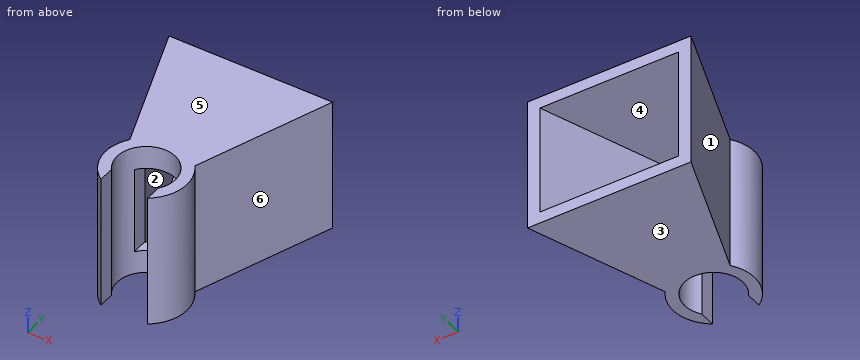
```python
from build123d import *

# Parameters (mm, degrees)
F1_DEPTH = 23
F3_DEPTH = 2
F5_DEPTH = 2
F6_W     = 8
F6_H     = 15
F7_DEPTH = 25


with BuildPart() as f1:
    # F0 (on Top) → F1 (new body)
    with BuildSketch(Plane.XY):
        with BuildLine():
            Line((-14.0209387689, 27.4292568356), (-5.5771887097, 4.2302442124))
            ThreePointArc((-5.5771887097, 4.2302442124), (-4.8480847739, 5.0493637247), (-4, 5.7445626465))
            Line((-4, 5.7445626465), (-11.892583224, 27.4292568356))
            Line((-11.892583224, 27.4292568356), (-14.0209387689, 27.4292568356))
        make_face()
        with BuildLine():
            ThreePointArc((-4, -3), (0, 5), (4, -3))
            Line((4, -3), (4, -5.7445626465))
            ThreePointArc((4, -5.7445626465), (6.9141036197, -1.0932388287), (5.5771887097, 4.2302442124))
            ThreePointArc((5.5771887097, 4.2302442124), (4.8480847739, 5.0493637247), (4, 5.7445626465))
            ThreePointArc((4, 5.7445626465), (0, 7), (-4, 5.7445626465))
            ThreePointArc((-4, 5.7445626465), (-4.8480847739, 5.0493637247), (-5.5771887097, 4.2302442124))
            ThreePointArc((-5.5771887097, 4.2302442124), (-6.9141036197, -1.0932388287), (-4, -5.7445626465))
            Line((-4, -5.7445626465), (-4, -3))
        make_face()
        with BuildLine():
            ThreePointArc((4, 5.7445626465), (4.8480847739, 5.0493637247), (5.5771887097, 4.2302442124))
            Line((5.5771887097, 4.2302442124), (14.0209387689, 27.4292568356))
            Line((14.0209387689, 27.4292568356), (11.892583224, 27.4292568356))
            Line((11.892583224, 27.4292568356), (4, 5.7445626465))
        make_face()
    extrude(amount=F1_DEPTH)

    # F2 (on face) → F3 (join)
    with BuildSketch(Plane.XY.offset(23)):
        with BuildLine():
            Line((11.892583224, 27.4292568356), (-11.892583224, 27.4292568356))
            Line((-11.892583224, 27.4292568356), (-4, 5.7445626465))
            ThreePointArc((-4, 5.7445626465), (0, 7), (4, 5.7445626465))
            Line((4, 5.7445626465), (11.892583224, 27.4292568356))
        make_face()
    extrude(amount=-F3_DEPTH)

    # F4 (on face) → F5 (join)
    with BuildSketch(Plane(origin=(0, 0, 0), x_dir=(1, 0, 0), z_dir=(0, 0, -1))):
        with BuildLine():
            Line((-11.892583224, -27.4292568356), (11.892583224, -27.4292568356))
            Line((11.892583224, -27.4292568356), (4, -5.7445626465))
            ThreePointArc((4, -5.7445626465), (0, -7), (-4, -5.7445626465))
            Line((-4, -5.7445626465), (-11.892583224, -27.4292568356))
        make_face()
    extrude(amount=-F5_DEPTH)

    # F6 (on Front) → F7 (cut)
    with BuildSketch(Plane.XZ):
        with Locations((0, 11.5)):
            Rectangle(F6_W, F6_H)
    extrude(amount=-F7_DEPTH, mode=Mode.SUBTRACT)


solid = f1.part
```
For this review, take the finished solid that the model builds, in its own axes (mm). Face numbers are marked on the shaded views. A direction names the side the tool comes from. Give positions to 0.01 mm unless a question says otherwise; leave off trailing zeros. Write each loop counter-clockwise with the first axis right and the second up, starting at its lowest first coordinate (ties: lowest second). Pieces come first, ordered by that corner, then holes. Notation, with made-up numbers: M -28.75,-14.5 L 8.25,-14.5 A28 cw 8.25,7.5 Z; hole C 79.5,89.25 d7. An arc over 180 degrees is marked long. One line per item, written item: value.
1) Take a section at B-B, the plane x = 0. Write out the cut boundary in (y, z).
Results are:
outline: M 5,0 L 27.43,0 L 27.43,2 L 7,2 L 7,4 L 5,4 Z; M 5,19 L 7,19 L 7,21 L 27.43,21 L 27.43,23 L 5,23 Z
2) Take a section at C-C, the plane z = 13.5. Write out the cut boundary in (x, y), then the cut area to 3 significant figures.
Results are:
outline: M -14.02,27.43 L -5.58,4.23 A7 ccw -4,-5.74 L -4,-3 A5 cw -4,3 L -4,5.74 L -11.89,27.43 Z; M 4,-5.74 A7 ccw 5.58,4.23 L 14.02,27.43 L 11.89,27.43 L 4,5.74 L 4,3 A5 cw 4,-3 Z
area: 135 mm²
3) For the marked faces 4, 5 and 6, list the 3-axis set-ups (+Z, -Z, +X, -X, +Y, -Y) from which the entire face can be reached by the end or side of a thin tool; tool diameter is ignored.
Results are:
face 4: +Y
face 5: +Z, +X, -X, +Y, -Y
face 6: +Z, -Z, +X
4) Take a section at A-A, the plane y = 0. Write out the cut boundary in (x, z), then the cut area to 3 significant figures.
Results are:
outline: M -7,0 L -5,0 L -5,23 L -7,23 Z; M 5,0 L 7,0 L 7,23 L 5,23 Z
area: 92.0 mm²
5) For line 1 (X direction, y = 4, z = 2.25); line 2 (X direction, y = 0, z = 5.25); line 3 (Z direction, x = 4.75, y = 26), list the stretches that pass through material, from the lowest coordinate up. Write a range as from..to.
Results are:
line 1: x = -5.74..-3, 3..5.74
line 2: x = -7..-5, 5..7
line 3: z = 0..2, 21..23
6) The part is to be moulded in two halves that separate along Z. For the marked faces 1, 2 and 3, say which applies: +Z half, -Z half, draft (parallel to the pull), parting line (faces both ways), or undercut.
Results are:
face 1: draft
face 2: undercut
face 3: -Z half
7) For P1, Ø8, axis at y = 23.5, z = 3.5, coming from the -X side; P2, Ø2, axis at y = -4, z = 17, coming from the +X side; P3, Ø0.8, axis at y = 4, z = 10, coming from the +X side; P4, Ø8, axis at x = 0, y = 0, coming from the -Z side, all flat-tipped, find the tip position at first contact; note any pin that passes through.
Results are:
P1: stops at x = -14.02
P2: stops at x = 6.32
P3: stops at x = 6
P4: passes through
8) Take a section at D-D, the plane z = 1.5. Write out the cut boundary in (x, y).
Results are:
outline: M -14.02,27.43 L -5.58,4.23 A7 ccw -4,-5.74 L -4,-3 A5 cw long 4,-3 L 4,-5.74 A7 ccw 5.58,4.23 L 14.02,27.43 Z
